Input: dimensioned drawing with shaded views. Units: mm. Origin: part minimum x, y, z. Round coordinates to 2 decimals unless told otherwise and drop trailing zeros. Loops run counter-clockwise (first coordinate to the right, second up) from the corner with the lowest first, then second, coordinate; pieces in that order, holes last.
Item 1: Section query A-A on x = 15. Return loops of the section in (y, z).
Item 2: Ray query, L1, parallel to Y at x = 95, z = 1.15; L2, parallel to Y at x = 95, z = 3.6. Return the intervals inside material, ascending.
Item 3: First-contact query: P1, Ø6.5, axis at x = 15, y = 115, coming from the +Z side; P2, Ø4.5, axis at x = 95, y = 115, coming from the +Z side. Flat tips, straight axial feed; report the tip coordinate or a pass-through.
Item 4: Section query C-C on y = 15. Return loops of the section in (x, z), then the cut area to 3 significant figures.
Item 5: Section query B-B on z = 2.75. Return loops of the section in (x, y).
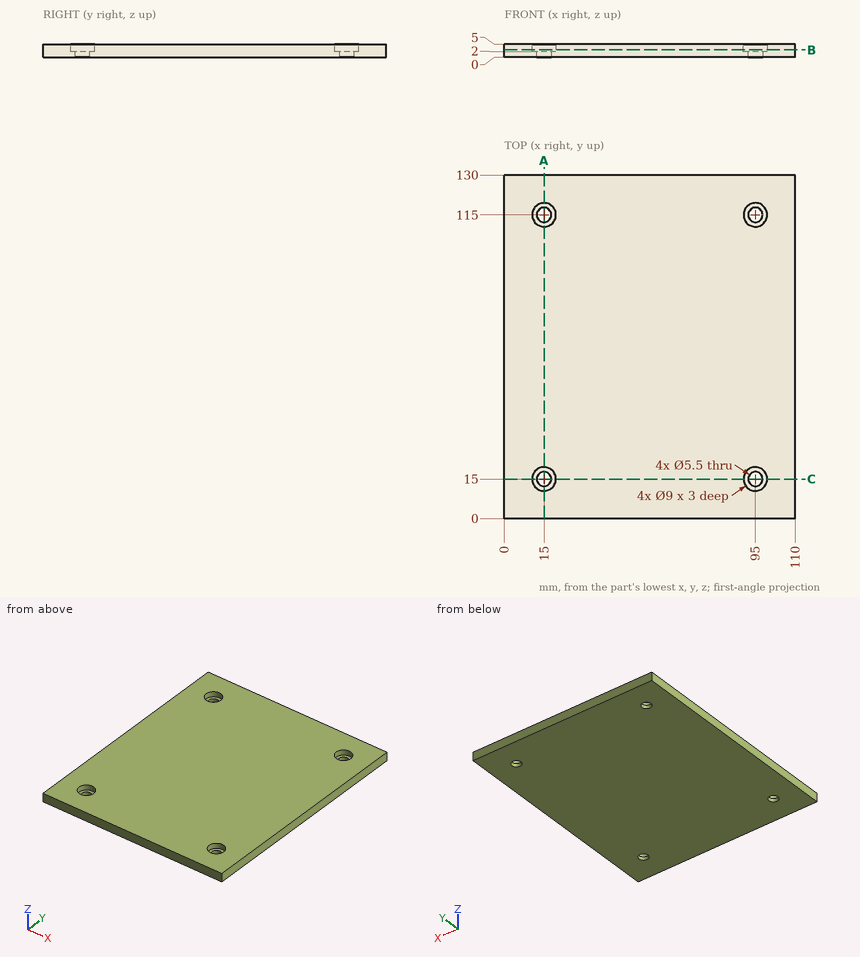
Data:
1. outline: (0, 0) - (12.25, 0) - (12.25, 2) - (10.5, 2) - (10.5, 5) - (0, 5) - close; (17.75, 0) - (112.25, 0) - (112.25, 2) - (110.5, 2) - (110.5, 5) - (19.5, 5) - (19.5, 2) - (17.75, 2) - close; (117.75, 0) - (130, 0) - (130, 5) - (119.5, 5) - (119.5, 2) - (117.75, 2) - close
2. L1: y = 0 to 12.25, 17.75 to 112.25, 117.75 to 130
2. L2: y = 0 to 10.5, 19.5 to 110.5, 119.5 to 130
3. P1: stops at z = 2
3. P2: passes through
4. outline: (0, 0) - (12.25, 0) - (12.25, 2) - (10.5, 2) - (10.5, 5) - (0, 5) - close; (17.75, 0) - (92.25, 0) - (92.25, 2) - (90.5, 2) - (90.5, 5) - (19.5, 5) - (19.5, 2) - (17.75, 2) - close; (97.75, 0) - (110, 0) - (110, 5) - (99.5, 5) - (99.5, 2) - (97.75, 2) - close
4. area: 474 mm2
5. outline: (0, 0) - (110, 0) - (110, 130) - (0, 130) - close; hole circle Ø9 at (15, 15); hole circle Ø9 at (15, 115); hole circle Ø9 at (95, 15); hole circle Ø9 at (95, 115)
